The listing builds one solid part. Answer for the finished solid, in the listing's coordinates (mm). A direction names the side the tool comes from. Give positions to 0.01 mm unless a question says otherwise; leave off trailing zeros. Order: outer loops, then holes, each group sorted by start corner. A loop starts at its lowest first (then second) coordinate and runs counter-clockwise, first axis right, second up. Notation, with made-up numbers: (-29.75, 36) - (2.25, 36) arc R30 cw to (2.25, 70) - close; hole circle Ø8 at (-12.5, -19). An arc over 180 degrees is marked (long way). Use a Markdown table: item, result. Add a question column.
1) For faces 5 (the face through (1.588, 2, -4)), 6 (the face through (7.271, 2, -4)), 7 (the face through (2, 2, -6.35)), 8 (the face through (11, 2, -1.588)), 9 (the face through (12.4, -1.79, -4.02)), determine the directions among +Z, -Z, +X, -X, +Y, -Y from which every point of the face is accessible in a straight line to the end or side of a thin tool.
2) Flat-ended cylindrical pins translate along their axes: pin 1 (0.8 mm diameter, centred on x = 6.5, y = 1.5, fed in from -Z); pin 2 (1.5 mm diameter, centred on y = 2.5, z = -6.5, fed in from -X); pin 3 (2.5 mm diameter, centred on y = 1.5, z = -4, fed in from +X). Find the tip coordinate at first contact, or state that the pin passes through.
3) Find section A-A, the plane y = 0.5. State how many separate pieces and enclosed holes the cut face has, plus the area to 3 significant figures.
4) Find section D-D, the plane y = -1.75. Determine the outline of the cut face in (x, z).
5) Straight lines are drawn through the part: line 1 (X direction, y = 0.5, z = -5.25) (1 decimal); line 2 (Z direction, x = 2.75, y = 1); line 3 (Z direction, x = 5.5, y = -2). For each, find the intervals that lie inside material, in ascending order.
6) The mould has two halves that part along X. Classify faces 1 (the face through (6, -3.175, -4)), 2 (the face through (3.175, 2, -4)), 3 (the face through (11.366, 2, -4)), 4 (the face through (0.554, -1.792, -4.024)): released by +X, released by -X, zero draft, split by the parting line, or undercut.
from build123d import *

# Parameters (mm, degrees)
SKETCH1_W           = 12.954
SKETCH1_H           = 7.9375
SKETCH1_W_2         = 1.5875
SKETCH1_H_2         = 4.7625
BOSS_EXTRUDE1_DEPTH = 3.175
SKETCH1_3_W         = 1.5875
SKETCH1_3_H         = 4.7625
BOSS_EXTRUDE2_DEPTH = 3.175
FILLET1_R           = 3.175


with BuildPart() as part:
    # Sketch1 → Boss-Extrude1 (new body)
    # profile 1 of 4: a face of its own
    with BuildSketch(Plane(origin=(0, 0, 0), x_dir=(1, 0, 0), z_dir=(0, 1, 0))):
        with Locations((6.477, 3.96875)):
            Rectangle(SKETCH1_W, SKETCH1_H)
        with Locations((10.57275, 3.96875)):
            Rectangle(SKETCH1_W_2, SKETCH1_H_2, mode=Mode.SUBTRACT)
        with Locations((6.477, 3.96875)):
            Rectangle(SKETCH1_W_2, SKETCH1_H_2, mode=Mode.SUBTRACT)
        with Locations((2.38125, 3.96875)):
            Rectangle(SKETCH1_W_2, SKETCH1_H_2, mode=Mode.SUBTRACT)
    # profile 2 of 4: a face of its own
    with BuildSketch(Plane(origin=(0, 0, 0), x_dir=(1, 0, 0), z_dir=(0, 1, 0))):
        with Locations((2.38125, 3.96875)):
            Rectangle(SKETCH1_W_2, SKETCH1_H_2)
    # profile 3 of 4: a face of its own
    with BuildSketch(Plane(origin=(0, 0, 0), x_dir=(1, 0, 0), z_dir=(0, 1, 0))):
        with Locations((6.477, 3.96875)):
            Rectangle(SKETCH1_W_2, SKETCH1_H_2)
    # profile 4 of 4: a face of its own
    with BuildSketch(Plane(origin=(0, 0, 0), x_dir=(1, 0, 0), z_dir=(0, 1, 0))):
        with Locations((10.57275, 3.96875)):
            Rectangle(SKETCH1_W_2, SKETCH1_H_2)
    extrude(amount=-BOSS_EXTRUDE1_DEPTH)

    # Sketch1<3> → Boss-Extrude2 (add)
    with BuildSketch(Plane(origin=(0, 0, 0), x_dir=(1, 0, 0), z_dir=(0, 1, 0))):
        with Locations((2.38125, 3.96875)):
            Rectangle(SKETCH1_3_W, SKETCH1_3_H)
        with Locations((6.477, 3.96875)):
            Rectangle(SKETCH1_3_W, SKETCH1_3_H)
        with Locations((10.57275, 3.96875)):
            Rectangle(SKETCH1_3_W, SKETCH1_3_H)
    extrude(amount=BOSS_EXTRUDE2_DEPTH)

    # Fillet1
    fillet1_edges = [part.edges().sort_by_distance(p)[0] for p in [
        (12.954, -3.175, -3.96875),
        (6.477, -3.175, -7.9375),
        (0, -3.175, -3.96875),
        (6.477, -3.175, 0),
    ]]
    fillet(fillet1_edges, radius=FILLET1_R - 0.0001)  # a hair under: the kernel refuses the full size


solid = part.part
The answers:
| question | item | result |
|---|---|---|
| 1 | face 5 | +Z, -Z, -X, +Y |
| 1 | face 6 | +Z, -Z, +Y |
| 1 | face 7 | -Z, +X, -X, +Y |
| 1 | face 8 | +Z, +X, -X, +Y |
| 1 | face 9 | +Z, -Z, +X, -Y |
| 2 | pin 1 | z = -6.35 |
| 2 | pin 2 | x = 1.59 |
| 2 | pin 3 | x = 11.37 |
| 3 | separate pieces | 3 |
| 3 | enclosed holes | 0 |
| 3 | area | 22.7 mm2 |
| 4 | outline | (0.53, -7.41) - (12.43, -7.41) - (12.43, -0.53) - (0.53, -0.53) - close |
| 5 | line 1 | 1.6 to 3.2, 5.7 to 7.3, 9.8 to 11.4 |
| 5 | line 2 | -6.35 to -1.59 |
| 5 | line 3 | -7.23 to -0.71 |
| 6 | face 1 | zero draft |
| 6 | face 2 | undercut |
| 6 | face 3 | released by +X |
| 6 | face 4 | released by -X |
